For this review, use the dimensioned drawing (mm, ordinates from the lowest corner) and the shaded views. Round coordinates to 2 decimals unless told otherwise and drop trailing zeros. Write each loop counter-clockwise with the first axis right and the second up, starting at its lowest first coordinate (ties: lowest second). Pieces come first, ordered by that corner, then holes. Notation, with made-up numbers: M 77.25,22.5 L 107.25,22.5 A19 cw 107.25,29.5 Z; hole C 41,57 d11. An arc over 180 degrees is marked long. Write each question's results on one line, items separated by ' | '. Start each with the question number.
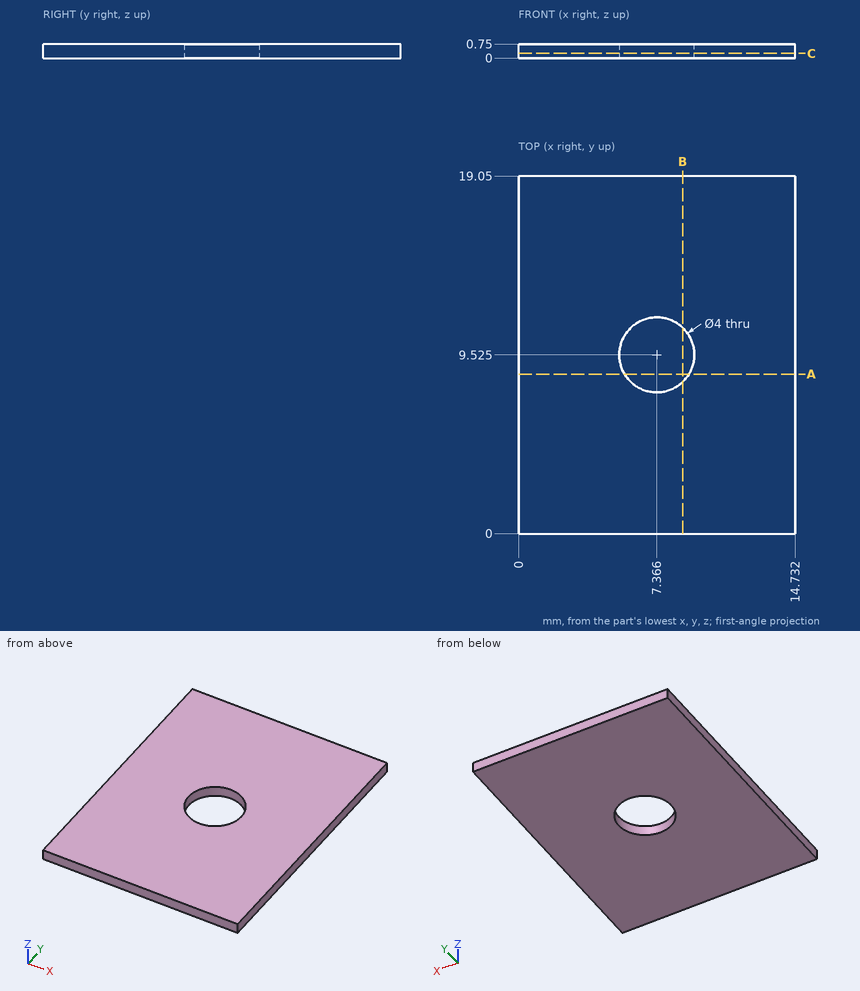
Item 1: We need section A-A on y = 8.5. State the section outline as (x, z) points, then the cut area to 3 significant figures.
Item 2: We need section C-C on z = 0.25. State the section outline as (x, y) points (3 decimals).
Item 3: For probe 1 along Y at (x, z) = (6.25, 0.7); probe 2 along Y at (x, z) = (8.25, 0.25); probe 3 along X at (y, z) = (8.75, 0.35), list the stretches that pass through material, from the lowest coordinate up.
Item 4: We need section B-B on x = 8.75. State the section outline as (y, z) points.
Numbers:
1) outline: M 0,0 L 5.65,0 L 5.65,0.75 L 0,0.75 Z; M 9.08,0 L 14.73,0 L 14.73,0.75 L 9.08,0.75 Z | area: 8.47 mm^2
2) outline: M 0,0 L 14.732,0 L 14.732,19.05 L 0,19.05 Z; hole C 7.366,9.525 d4
3) probe 1: y = 0 to 7.87, 11.18 to 19.05 | probe 2: y = 0 to 7.73, 11.32 to 19.05 | probe 3: x = 0 to 5.52, 9.21 to 14.73
4) outline: M 0,0 L 8.08,0 L 8.08,0.75 L 0,0.75 Z; M 10.97,0 L 19.05,0 L 19.05,0.75 L 10.97,0.75 Z
